Here's the drawing with two shaded views (mm, measured from the low corner). I have some questions. A direction names the side the tool comes from. Give positions to 0.01 mm unless a question says otherwise; leave off trailing zeros. Write each loop counter-clockwise with the first axis right and the second up, starting at its lowest first coordinate (ties: lowest second). Pieces come first, ordered by that corner, then holes. Notation, with made-up numbers: (-8.5, 43.25) - (27.5, 43.25) arc R30 cw to (27.5, 76.25) - close; hole circle Ø2 at (6, 1.5). An arc over 180 degrees is marked (long way). Answer as CSV lines item,"result". Start each with the question number.
Q1. Imagine slicing it at C-C on x = 12.5. List the corners of the cut face in (y, z) for me, and give its area (3 significant figures).
Q2. Imagine slicing it at A-A on y = 15. List the corners of the cut face in (x, z) for me.
Q3. If I drill on line 1 along Y through (x, z) = (11.8, 15); line 2 along Z through (x, y) = (3.75, 15); line 3 along X through (y, z) = (21.25, 9.25), over which ranges is the centre line in solid material (lowest first)?
Q4. Imagine slicing it at D-D on x = 3.5. List the corners of the cut face in (y, z) for me.
Q5. Imagine slicing it at B-B on z = 15. List the corners of the cut face in (x, y) for me.
Q6. On a 3-axis mill with a long thin cutter (end or side, diameter ignored), from which of +Z, -Z, +X, -X, +Y, -Y can I reach the whole of each face in a straight line? I mean the marked faces 1 and 2. Say none if no direction works.
Q7. Will these pins go through, and if not, where does the flat tip stop? pin 1 Ø5 at (y, z) = (4, 14.5) entering from -X; pin 2 Ø2.5 at (y, z) = (10, 6.34) entering from +X (1 decimal); pin 3 Ø1.5 at (x, y) = (12.5, 8) entering from +Z.
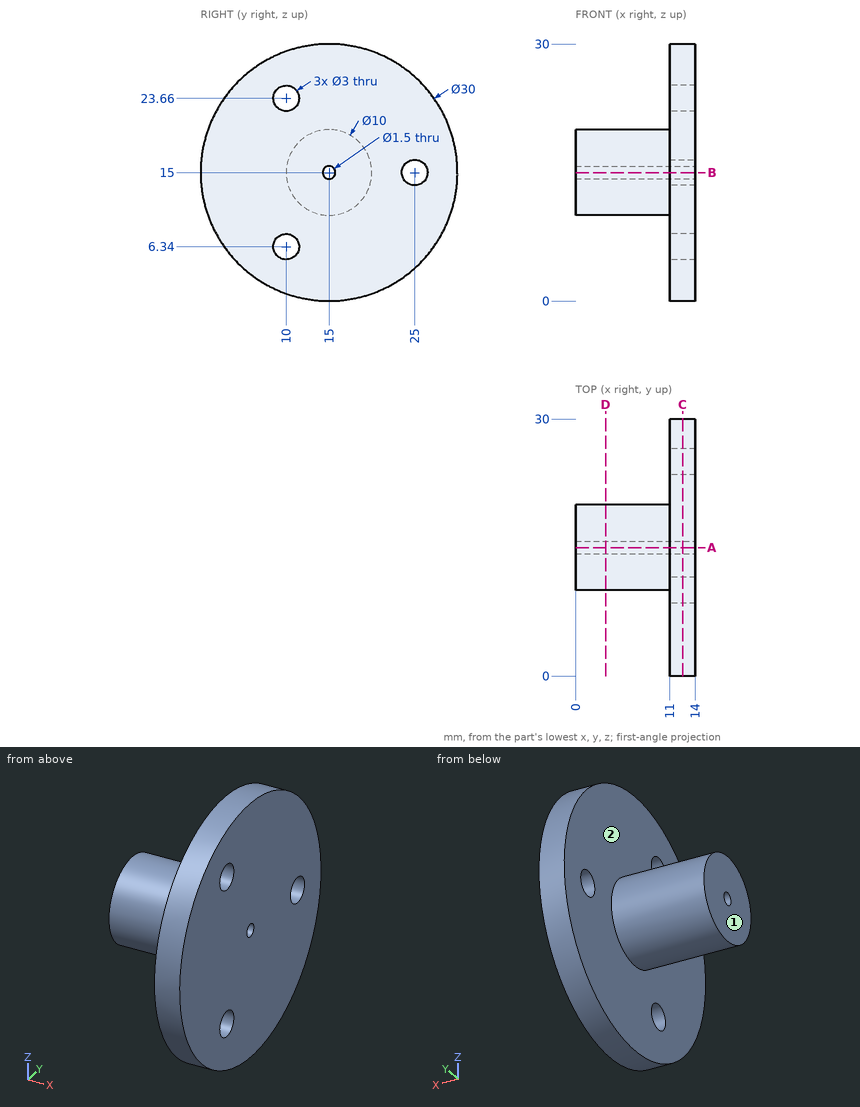
Conclusion:
1,outline,"circle Ø30 at (15, 15); hole circle Ø3 at (10, 6.34); hole circle Ø3 at (10, 23.66); hole circle Ø1.5 at (15, 15); hole circle Ø3 at (25, 15)"
1,area,"684 mm^2"
2,outline,"(0, 10) - (11, 10) - (11, 0) - (14, 0) - (14, 14.25) - (0, 14.25) - close; (0, 15.75) - (14, 15.75) - (14, 30) - (11, 30) - (11, 20) - (0, 20) - close"
3,line 1,"0 to 14.25, 15.75 to 23.5, 26.5 to 30"
3,line 2,"10 to 14.25, 15.75 to 20"
3,line 3,"11 to 14"
4,outline,"circle Ø10 at (15, 15); hole circle Ø1.5 at (15, 15)"
5,outline,"(0, 10) - (11, 10) - (11, 0) - (14, 0) - (14, 14.25) - (0, 14.25) - close; (0, 15.75) - (14, 15.75) - (14, 23.5) - (11, 23.5) - (11, 20) - (0, 20) - close; (11, 26.5) - (14, 26.5) - (14, 30) - (11, 30) - close"
6,face 1,"+Z, -Z, -X, +Y, -Y"
6,face 2,"-X"
7,pin 1,"x = 11"
7,pin 2,"through"
7,pin 3,"z = 28.64"
